Can you work these out from the drawing? Everything is in mm from the part's minimum corner. Give positions to 0.01 mm unless a question says otherwise; leave off trailing zeros. Order: outer loops, then holes, each group sorted by start corner. A loop starts at its lowest first (then second) coordinate and runs counter-clockwise, first axis right, second up. Notation, with made-up numbers: M 43.25,8.5 L 82.25,8.5 A32 ccw 82.25,38.5 Z; hole C -1,81 d7. An arc over 180 degrees is marked long. Answer in a Markdown table with one row per item. Add a question column.
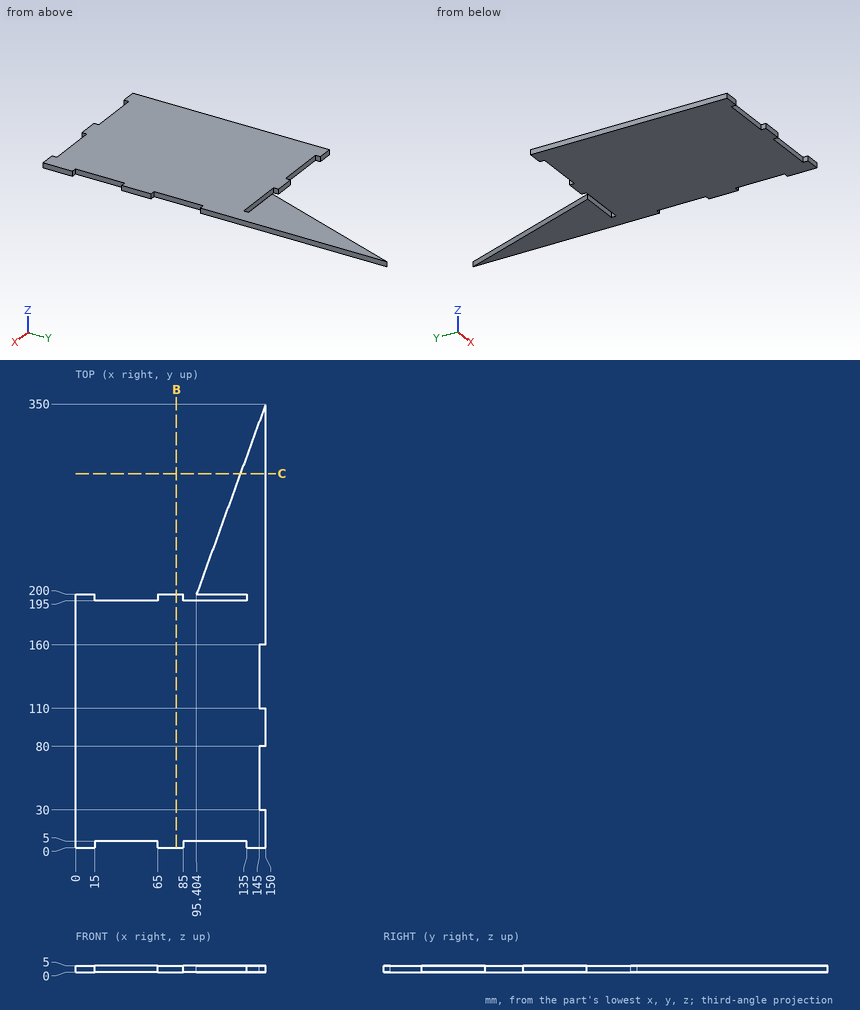
1. If I drill on line 1 along X through (y, z) = (45, 0.4); line 2 along Y through (x, z) = (35, 3.15); line 3 along Y through (x, z) = (80, 1.45), over which ranges is the centre line in solid material (lowest first)? Write a range as [from, to].
2. Suppose I cut it at B-B on x = 79.5. List the corners of the cut face in (y, z) for me, plus the area to 3 significant figures.
3. Suppose I cut it at C-C on y = 295. List the corners of the cut face in (x, z) for me, plus the area to 3 significant figures.
4. Will these pins go through, and if not, where does the flat tip stop? P1, Ø2, axis at x = 83, z = 0.5, coming from the +Y side; P2, Ø1.5, axis at y = 56, z = 1.5, coming from the +X side; P3, Ø2.5, axis at x = 44.5, z = 1.5, coming from the -Y side.
Findings below:
| question | item | result |
|---|---|---|
| 1 | line 1 | [0, 145] |
| 1 | line 2 | [5, 195] |
| 1 | line 3 | [0, 200] |
| 2 | outline | M 0,0 L 200,0 L 200,5 L 0,5 Z |
| 2 | area | 1,000 mm2 |
| 3 | outline | M 129.98,0 L 150,0 L 150,5 L 129.98,5 Z |
| 3 | area | 100 mm2 |
| 4 | P1 | y = 200 |
| 4 | P2 | x = 145 |
| 4 | P3 | y = 5 |
